from build123d import *

# Parameters (mm, degrees)
F0_W           = 48
F0_H           = 106
F1_DEPTH       = 7.5
F4_DEPTH       = 25
F6_D           = 5.5
F6_CBORE_D     = 8
F6_CBORE_DEPTH = 6


with BuildPart() as f1:
    # F0 (on Top) → F1 (new body, symmetric)
    with BuildSketch(Plane.XY):
        with Locations((9.722433, 20.829119)):
            Rectangle(F0_W, F0_H)
    extrude(amount=F1_DEPTH, both=True)

    # F3 (on face) → F4 (join)
    with BuildSketch(Plane.XY.offset(7.5)):
        Polygon((-6.277567, 20.829119), (-6.277567, 73.829119), (-14.277567, 73.829119), (-14.277567, -32.170881), (-6.277567, -32.170881), align=None)
        Polygon((33.722433, 73.829119), (25.722433, 73.829119), (25.722433, 20.829119), (25.722433, -32.170881), (33.722433, -32.170881), align=None)
    extrude(amount=F4_DEPTH)

    # F6 (through all)
    with Locations(Plane.XY.offset(7.5)):
        with Locations((9.722433, 40.829119), (9.722433, 60.829119), (9.722433, 2.829119), (9.722433, -17.170881)):
            CounterBoreHole(F6_D / 2, F6_CBORE_D / 2, F6_CBORE_DEPTH)


solid = f1.part
Here's how the part is built. I have some questions about the finished solid (model axes, mm). A direction names the side the tool comes from. Round coordinates to 2 decimals unless told otherwise and drop trailing zeros. Order: outer loops, then holes, each group sorted by start corner. A loop starts at its lowest first (then second) coordinate and runs counter-clockwise, first axis right, second up. Notation, with made-up numbers: (-23, -14) -> (-13, -14) arc R18 ccw to (-13, 16) -> close; hole circle Ø11 at (14.5, -34). An arc over 180 degrees is marked (long way). Use CSV: the item, a comma, the result in double quotes.
1. I'm going to push a flat-ended pin straight in: P1, Ø5, axis at x = -1.5, y = 10, coming from the +Z side. Where does the tip first touch, or does it pass through?
Recorded:
P1,"stops at z = 7.5"
2. I want a section at A-A on z = 24. List the corners of the cut face in (x, y) for me, and give its area (3 significant figures).
Recorded:
outline,"(-14.28, -32.17) -> (-6.28, -32.17) -> (-6.28, 73.83) -> (-14.28, 73.83) -> close; (25.72, -32.17) -> (33.72, -32.17) -> (33.72, 73.83) -> (25.72, 73.83) -> close"
area,"1,700 mm2"
3. Thinking about a two-plate mould opening in X: for faces 4 (the face through (9, -32.171, 3)), 5 (the face through (33.722, 20, 13)), 6 (the face through (13.42, 1.3, 4.54)), which applies, pulls with the +X half, pulls with the -X half, needs draft (parallel to the pull), parting line crosses it, or undercut?
Recorded:
face 4,"needs draft"
face 5,"pulls with the +X half"
face 6,"undercut"
4. Which directions (+Z, -Z, +X, -X, +Y, -Y) give clear straight access to the entire face, cutting with the end or side of a thin tool? Please do faces 1 (the face through (9, 58, 1.5)), 2 (the face through (9, 22, 7.5)), 3 (the face through (30, 22, 32.5)).
Recorded:
face 1,"+Z"
face 2,"+Z, +Y, -Y"
face 3,"+Z, +X, -X, +Y, -Y"
5. I need wall thicknesses on line 1 along X through (y, z) = (26, 22); line 2 along Y through (x, z) = (8, -2.5); line 3 along Z through (x, y) = (13, 2). Which ranges of each line are inside material? Lowest first, please.
Recorded:
line 1,"x = -14.28 to -6.28, 25.72 to 33.72"
line 2,"y = -32.17 to -19.31, -15.03 to 0.69, 4.97 to 38.69, 42.97 to 58.69, 62.97 to 73.83"
line 3,"z = -7.5 to 1.5"
6. I want a section at B-B on y = 47.5. List the corners of the cut face in (x, z) for me.
Recorded:
outline,"(-14.28, -7.5) -> (33.72, -7.5) -> (33.72, 32.5) -> (25.72, 32.5) -> (25.72, 7.5) -> (-6.28, 7.5) -> (-6.28, 32.5) -> (-14.28, 32.5) -> close"
7. I want a section at D-D on x = -1. List the corners of the cut face in (y, z) for me, and give its area (3 significant figures).
Recorded:
outline,"(-32.17, -7.5) -> (73.83, -7.5) -> (73.83, 7.5) -> (-32.17, 7.5) -> close"
area,"1,590 mm2"
8. I want a section at C-C on z = 3. List the corners of the cut face in (x, y) for me.
Recorded:
outline,"(-14.28, -32.17) -> (33.72, -32.17) -> (33.72, 73.83) -> (-14.28, 73.83) -> close; hole circle Ø8 at (9.72, -17.17); hole circle Ø8 at (9.72, 2.83); hole circle Ø8 at (9.72, 40.83); hole circle Ø8 at (9.72, 60.83)"
